Study the drawing (mm; zero at the part's minimum x, y, z) and answer. A direction names the side the tool comes from. Coordinates: 2 decimals unless noted, no trailing zeros. Order: outer loops, then holes, each group sorted by start corner. A loop starts at its lowest first (then second) coordinate and runs counter-clockwise, first axis right, second up. Notation, with made-up numbers: M 41.25,3.5 L 91.25,3.5 A34 cw 91.25,36.5 Z; hole C 85.5,33.25 d6. An arc over 180 degrees is marked long. One line per item, written item: value. Start each with the question number.
Q1. Straight lines are drawn through the part: line 1 along Y through (x, z) = (7, 5.25); line 2 along X through (y, z) = (1.75, 9); line 3 along Y through (x, z) = (23, 11.5). For each, find the intervals that lie inside material, in ascending order. Write a range as [from, to].
Q2. Each of these flat-tipped pins is pushed along its axis until it touches: pin 1 Ø4 at (x, z) = (15, 15) entering from -Y; pin 2 Ø1.9 at (y, z) = (10.03, 10.51) entering from -X. Where does it stop, or does it pass through?
Q3. The part is cut by section C-C on z = 17. Give the vertices of the cut face in (x, y).
Q4. For the marked faces 1 and 2, determine the directions among +Z, -Z, +X, -X, +Y, -Y from which every point of the face is accessible in a straight line to the end or side of a thin tool.
Q5. The part is cut by section B-B on y = 25. Give the vertices of the cut face in (x, z).
Q6. The part is cut by section A-A on x = 6.5. Give the vertices of the cut face in (y, z) (3 decimals), then the cut area to 3 significant figures.
Q7. The part is cut by section D-D on y = 5.75. Give the vertices of the cut face in (x, z).
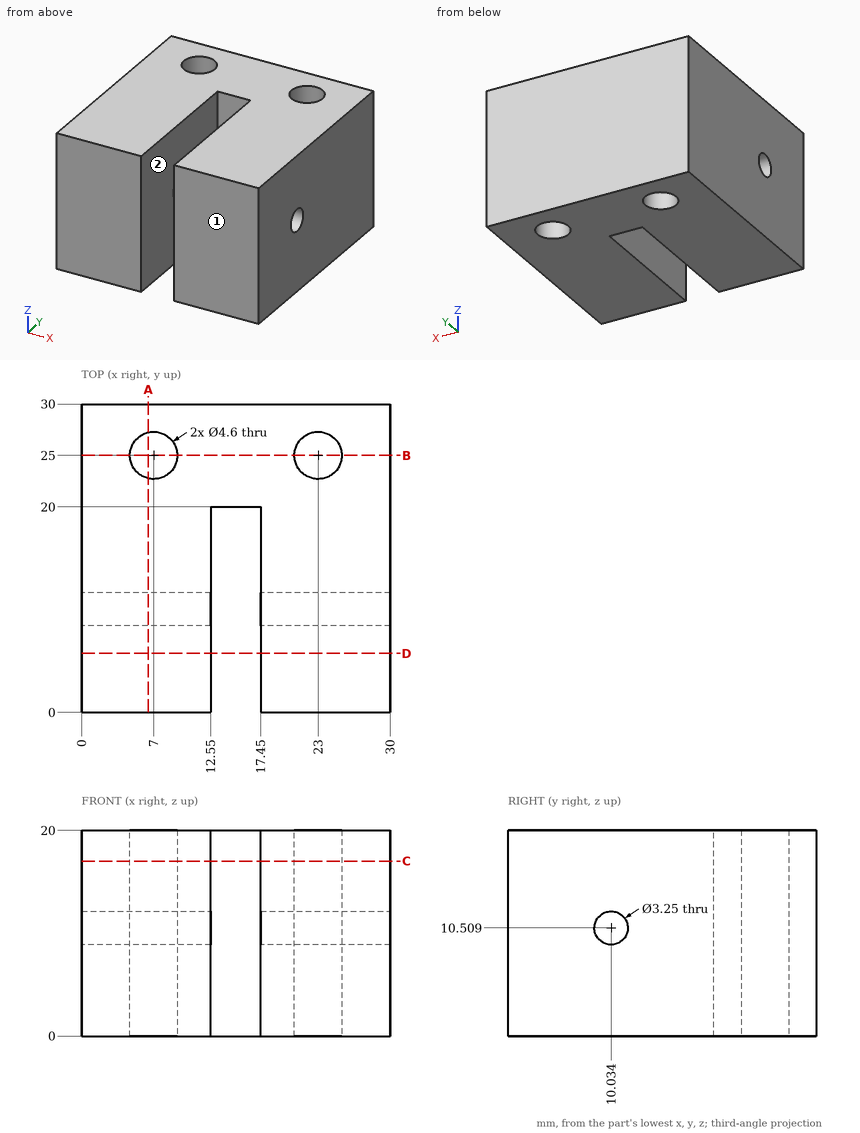
Output:
1. line 1: y = [0, 22.7], [27.3, 30]
1. line 2: x = [0, 12.55], [17.45, 30]
1. line 3: y = [0, 8.75], [11.32, 22.7], [27.3, 30]
2. pin 1: stops at y = 20
2. pin 2: passes through
3. outline: M 0,0 L 12.55,0 L 12.55,20 L 17.45,20 L 17.45,0 L 30,0 L 30,30 L 0,30 Z; hole C 7,25 d4.6; hole C 23,25 d4.6
4. face 1: +Z, -Z, +X, -X, -Y
4. face 2: +Z, -Z, -Y
5. outline: M 0,0 L 4.7,0 L 4.7,20 L 0,20 Z; M 9.3,0 L 20.7,0 L 20.7,20 L 9.3,20 Z; M 25.3,0 L 30,0 L 30,20 L 25.3,20 Z
6. outline: M 0,0 L 22.755,0 L 22.755,20 L 0,20 Z; M 27.245,0 L 30,0 L 30,20 L 27.245,20 Z; hole C 10.034,10.509 d3.25
6. area: 502 mm^2
7. outline: M 0,0 L 12.55,0 L 12.55,20 L 0,20 Z; M 17.45,0 L 30,0 L 30,20 L 17.45,20 Z
